```python
from build123d import *

# Parameters (mm, degrees)
SKETCH_1_R               = 7.5
EXTRUDE_1_DEPTH          = 5
EXTRUDE_START            = -3
SKETCH_2_R               = 7.5
SKETCH_2_R_2             = 2
EXTRUDE_2_DEPTH          = 3
EXTRUDE_3_DEPTH          = 12
EXTRUDE_3_DEPTH_BACK     = 15
SKETCH_3_R               = 32.5
SKETCH_3_R_2             = 22.5
REVOLVE_1_ANGLE          = 12
PATTERN_CIRCULAR_1_COUNT = 10
SKETCH_5_R               = 4.5
CUT_EXTRUDE_1_DEPTH      = 2
FILLET_1_R               = 1


with BuildPart() as part:
    # Sketch 1 → Extrude 1 (new body)
    with BuildSketch(Plane.XY):
        Circle(SKETCH_1_R)
        Polygon((-6.92820323, 0), (-3.464101615, -6), (3.464101615, -6), (6.92820323, 0), (3.464101615, 6), (-3.464101615, 6), align=None, mode=Mode.SUBTRACT)
    extrude(amount=EXTRUDE_1_DEPTH)

    # Sketch 2 → Extrude 2 (add)
    with BuildSketch(Plane.XY.offset(EXTRUDE_START)):
        Circle(SKETCH_2_R)
        Circle(SKETCH_2_R_2, mode=Mode.SUBTRACT)
    extrude(amount=EXTRUDE_2_DEPTH)



with BuildPart() as body_2:
    # Sketch 3 → Extrude 3 (new, two sides: drawn at the far end of the back side and taken through both)
    with BuildSketch(Plane.XY.offset(-EXTRUDE_3_DEPTH_BACK)):
        Circle(SKETCH_3_R)
        Circle(SKETCH_3_R_2, mode=Mode.SUBTRACT)
    extrude(amount=EXTRUDE_3_DEPTH + EXTRUDE_3_DEPTH_BACK)


with BuildPart() as part_1:
    add(part.part)

    add(body_2.part)  # Revolve 1 merges body 2
    # Sketch 4 → Revolve 1 (revolve)
    with BuildSketch(Plane(origin=(0, 0, 0), x_dir=(0, 0, -1), z_dir=(1, 0, 0))):
        Polygon((-5, 7.5), (3, 7.5), (15, 22.5), (7, 22.5), align=None)
    revolve_1 = revolve(axis=Axis((0, 0, -16.35), (0, 0, 1)), revolution_arc=REVOLVE_1_ANGLE)

    # Pattern Circular 1: Revolve 1 ×10 about axis
    pattern_circular_1_axis = Axis((0, 0, 0), (0, 0, 1))
    for i in range(1, PATTERN_CIRCULAR_1_COUNT):
        add(revolve_1.rotate(pattern_circular_1_axis, i * 360 / PATTERN_CIRCULAR_1_COUNT))

    # Sketch 5 → Cut-Extrude 1 (cut)
    with BuildSketch(Plane(origin=(0, 0, -3), x_dir=(-1, 0, 0), z_dir=(0, 0, -1))):
        Circle(SKETCH_5_R)
    extrude(amount=-CUT_EXTRUDE_1_DEPTH, mode=Mode.SUBTRACT)

    # Fillet 1
    fillet_1_edges = [part_1.edges().sort_by_distance(p)[0] for p in [
        (-32.5, 0, -15),
        (-32.5, 0, 12),
    ]]
    fillet(fillet_1_edges, radius=FILLET_1_R)


solid = part_1.part
```
CAD build for the part. Positions are in the model's coordinates, mm. A direction names the side the tool comes from. Give positions to 0.01 mm unless a question says otherwise; leave off trailing zeros. Loops run counter-clockwise (first coordinate to the right, second up) from the corner with the lowest first, then second, coordinate; pieces in that order, holes last. Notation, with made-up numbers: (-16, 0.25) -> (36, 0.25) arc R20 cw to (36, 23.25) -> close; hole circle Ø6 at (26, 3.5). An arc over 180 degrees is marked (long way). Use a Markdown table: item, result.
1. Wall check: L1, parallel to X at y = 17, z = -13.5; L2, parallel to Y at x = 11, z = 3.5; L3, parallel to Y at x = -7, z = -13.75. Give the ranges that are in metal, low to high. Write a range as [from, to].
Check result:
| item | result |
|---|---|
| L1 | x = [-27.7, -12.35], [11.68, 12.35], [14.74, 27.7] |
| L2 | y = [-30.58, -19.63], [19.63, 30.58] |
| L3 | y = [-31.74, -21.38], [21.38, 31.74] |
2. Flat gauge pins, fed straight in: pin 1 (3.5 mm diameter, centred on x = 0, y = 0, fed in from +Z); pin 2 (2.5 mm diameter, centred on x = 1.5, z = 3, fed in from +Y); pin 3 (8 mm diameter, centred on x = 0, y = 0, fed in from -Z); pin 4 (13 mm diameter, centred on x = -2.5, y = 0.5, fed in from +Z). Where does each tip first touch, or does it go through?
Check result:
| item | result |
|---|---|
| pin 1 | passes through |
| pin 2 | stops at y = 32.5 |
| pin 3 | stops at z = -1 |
| pin 4 | stops at z = 5 |
3. Slice it at A-A (z = 6.25). List the corners of the cut face in (x, y).
Check result:
| item | result |
|---|---|
| outline | circle Ø65 at (0, 0); hole circle Ø45 at (0, 0) |
4. Which spindle directions (+Z, -Z, +X, -X, +Y, -Y) get a long thin tool onto all of the face, cutting with end or side? Do faces 1 (the flat face through (0, -15, -5)), 2 (the flat face through (-21.44, 7.44, 12)), 3 (the conical face through (13.808, 6.124, -9.084)), 4 (the cylindrical face through (10.382, -19.961, -1.689)). Say none if no direction does.
Check result:
| item | result |
|---|---|
| face 1 | +Z, -Z |
| face 2 | +Z, +X, -X, +Y, -Y |
| face 3 | -Z |
| face 4 | +Z |
5. Slice it at B-B (x = 10.5). Give the number of separate pieces and of enclosed holes in the cut face, plus the area to 3 significant figures.
Check result:
| item | result |
|---|---|
| separate pieces | 5 |
| enclosed holes | 0 |
| area | 709 mm^2 |
